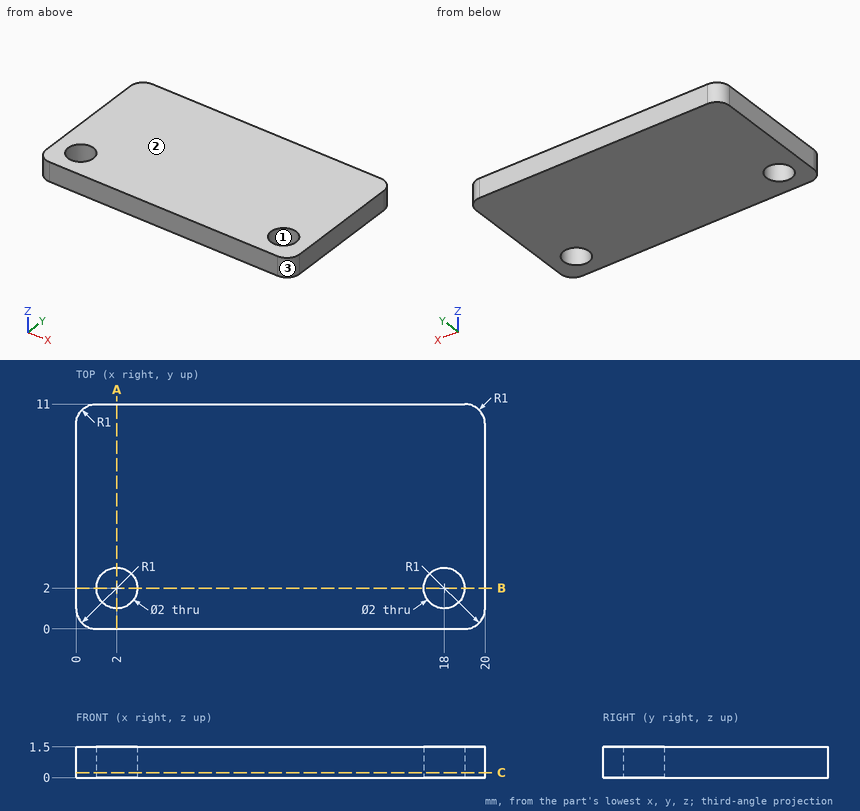
Input: dimensioned drawing with shaded views. Units: mm. Origin: part minimum x, y, z. Give positions to 0.01 mm unless a question says otherwise; leave off trailing zeros. Write each loop counter-clockwise with the first axis right and the second up, starting at its lowest first coordinate (ties: lowest second). Pieces come first, ordered by that corner, then holes. Notation, with made-up numbers: (65.5, 74.25) - (80.5, 74.25) arc R16 ccw to (80.5, 103.25) - close; hole circle Ø6 at (-35.5, 40.25). An arc over 180 degrees is marked (long way). Write item = value, one per line. Start each with the question number.
1) Draft query along Y for the marked faces 1, 2 and 3. Return one class per face: pulls with the +Y half, pulls with the -Y half, needs draft (parallel to the pull), parting line crosses it, or undercut.
2) Cut plane B-B (y = 2). Return loops of the section in (x, z), and give its area (3 significant figures).
3) Cut plane A-A (x = 2). Return loops of the section in (y, z), and give its area (3 significant figures).
4) Material intervals for L1, parallel to Y at x = 2, z = 1.15; L2, parallel to X at y = 1.5, z = 0.65; L3, parallel to Y at x = 1.25, z = 1.3, sorted ascending. Write a range as [from, to].
5) Cut plane C-C (z = 0.25). Return loops of the section in (x, y), and give its area (3 significant figures).
Answers follow:
q1.face_1 = undercut
q1.face_2 = needs draft
q1.face_3 = pulls with the -Y half
q2.outline = (0, 0) - (1, 0) - (1, 1.5) - (0, 1.5) - close; (3, 0) - (17, 0) - (17, 1.5) - (3, 1.5) - close; (19, 0) - (20, 0) - (20, 1.5) - (19, 1.5) - close
q2.area = 24.0 mm^2
q3.outline = (0, 0) - (1, 0) - (1, 1.5) - (0, 1.5) - close; (3, 0) - (11, 0) - (11, 1.5) - (3, 1.5) - close
q3.area = 13.5 mm^2
q4.L1 = [0, 1], [3, 11]
q4.L2 = [0, 1.13], [2.87, 17.13], [18.87, 20]
q4.L3 = [0, 1.34], [2.66, 11]
q5.outline = (0, 1) arc R1 ccw to (1, 0) - (19, 0) arc R1 ccw to (20, 1) - (20, 10) arc R1 ccw to (19, 11) - (1, 11) arc R1 ccw to (0, 10) - close; hole circle Ø2 at (2, 2); hole circle Ø2 at (18, 2)
q5.area = 213 mm^2
